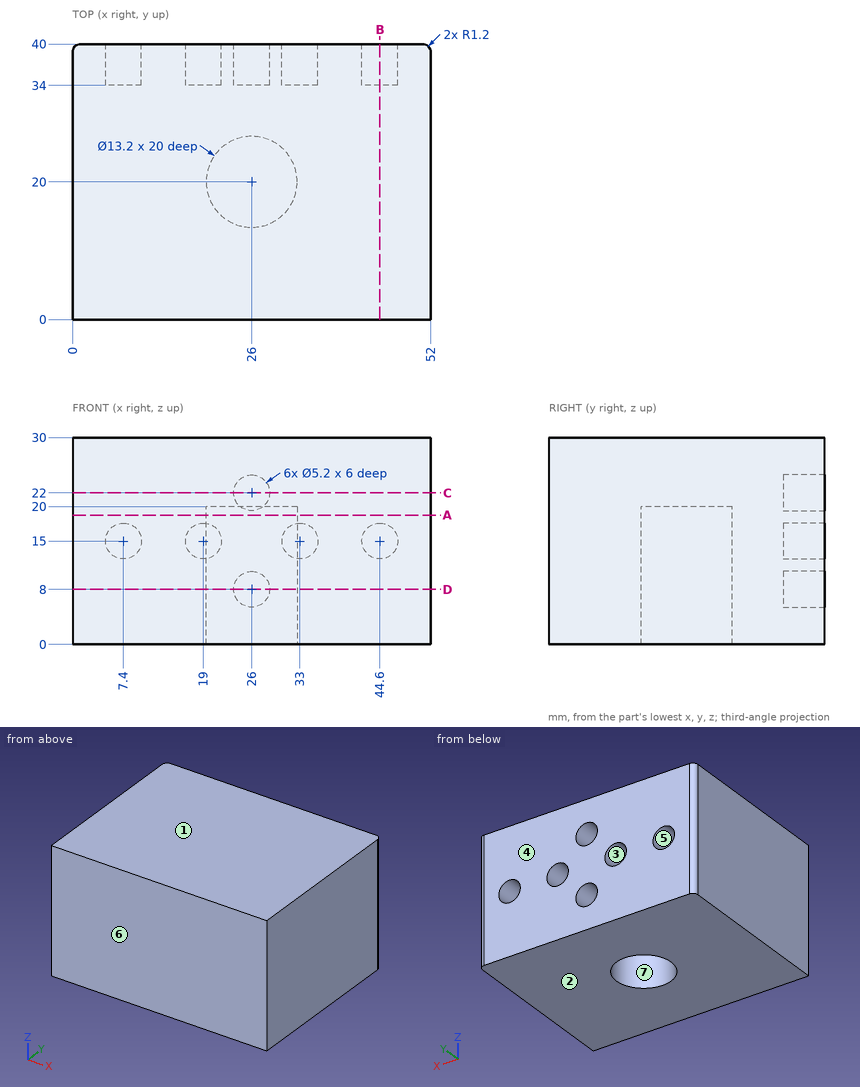
Input: dimensioned drawing with shaded views. Units: mm. Origin: part minimum x, y, z. A direction names the side the tool comes from. Round coordinates to 2 decimals unless told otherwise and drop trailing zeros. Loops run counter-clockwise (first coordinate to the right, second up) from the corner with the lowest first, then second, coordinate; pieces in that order, holes last. Notation, with made-up numbers: M 30,-15 L 51,-15 A27 cw 51,16 Z; hole C 76,7 d1. An arc over 180 degrees is marked long. One line per question, with ' | ' between items.
(1) Contact query for flat-ended pins moving along their axis: P1, Ø1.6, axis at x = 26.5, z = 21, coming from the +Y side; P2, Ø4, axis at x = 28, y = 17, coming from the -Z side. Output: stop coordinate, or through.
Check result:
P1: stops at y = 34 | P2: stops at z = 20
(2) Material intervals for line 1 along X through (y, z) = (37.25, 15); line 2 along Y through (x, z) = (26, 13.5); line 3 along X through (y, z) = (17, 16), sorted ascending. Write a range as from..to.
Check result:
line 1: x = 0..4.8, 10..16.4, 21.6..30.4, 35.6..42, 47.2..52 | line 2: y = 0..13.4, 26.6..40 | line 3: x = 0..20.12, 31.88..52
(3) Pull-direction query (Z, two-part tool) for the marked faces 1, 2, 3 and 4; classes: +Z half, -Z half, draft (parallel to the pull), parting line (faces both ways), or undercut.
Check result:
face 1: +Z half | face 2: -Z half | face 3: undercut | face 4: draft
(4) Cut plane A-A on z = 18.75. Return the cut outline in (x, y), plus the area to 3 significant figures.
Check result:
outline: M 0,0 L 52,0 L 52,38.8 A1.2 ccw 50.8,40 L 1.2,40 A1.2 ccw 0,38.8 Z; hole C 26,20 d13.2 | area: 1,940 mm2
(5) Cut plane C-C on z = 22. Return the cut outline in (x, y), plus the area to 3 significant figures.
Check result:
outline: M 0,0 L 52,0 L 52,38.8 A1.2 ccw 50.8,40 L 28.6,40 L 28.6,34 L 23.4,34 L 23.4,40 L 1.2,40 A1.2 ccw 0,38.8 Z | area: 2,050 mm2
(6) Access query for the marked faces 5, 6 and 7. Directions: +Z, -Z, +X, -X, +Y, -Y. A direction counts if a zero-diameter tool reaches every point of the face in a straight line with its end or side. Return the directions, or none.
Check result:
face 5: +Y | face 6: +Z, -Z, +X, -X, -Y | face 7: -Z
(7) Cut plane B-B on x = 44.6. Return the cut outline in (y, z), plus the area to 3 significant figures.
Check result:
outline: M 0,0 L 40,0 L 40,12.4 L 34,12.4 L 34,17.6 L 40,17.6 L 40,30 L 0,30 Z | area: 1,170 mm2
(8) Cut plane D-D on z = 8. Return the cut outline in (x, y).
Check result:
outline: M 0,0 L 52,0 L 52,38.8 A1.2 ccw 50.8,40 L 28.6,40 L 28.6,34 L 23.4,34 L 23.4,40 L 1.2,40 A1.2 ccw 0,38.8 Z; hole C 26,20 d13.2
